Part model, mm, in its own coordinate system. Face numbers are marked on the shaded views. A direction names the side the tool comes from. Round coordinates to 2 decimals unless told otherwise and drop trailing zeros. Write each loop counter-clockwise with the first axis right and the second up, starting at its lowest first coordinate (ties: lowest second). Pieces come first, ordered by that corner, then holes. Notation, with made-up numbers: (34.25, 60) -> (61.25, 60) arc R19 ccw to (61.25, 67) -> close; hole circle Ø9 at (86, -32.5). An arc over 180 degrees is marked (long way). Use CSV: the item, a comma, the result in double quotes. Start each with the question number.
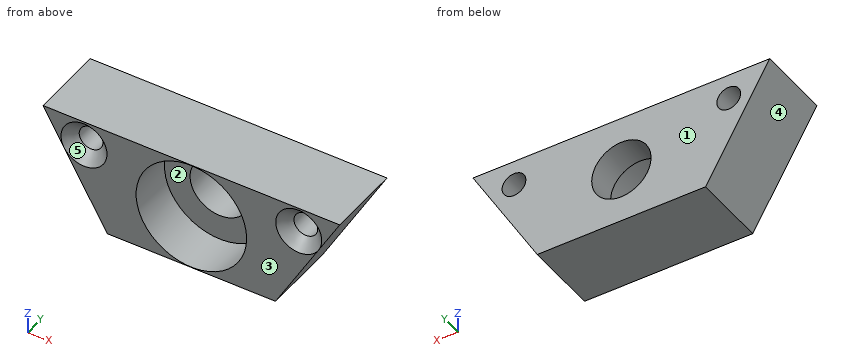
```python
from build123d import *

# Parameters (mm, degrees)
F0_R     = 1.6
F0_R_2   = 4
F1_DEPTH = 10
F2_R     = 7.45
F2_R_2   = 4
F3_DEPTH = 6


# Not quite as in the source:
# - a fillet or chamfer that OpenCascade refuses, or shapes differently, is made with other operations: its cross-section is extruded or revolved along the edge and cut away or added


with BuildPart() as f1:
    # F0 (on Front) → F1 (new body)
    with BuildSketch(Plane.XZ):
        Polygon((20, 7.5), (-20, 7.5), (-11.3397459622, -7.5), (11.3397459622, -7.5), align=None)
        with Locations((-14.4742550328, 4.1231745854)):
            Circle(F0_R, mode=Mode.SUBTRACT)
        Circle(F0_R_2, mode=Mode.SUBTRACT)
        with Locations((14.4742550328, 4.1231745854)):
            Circle(F0_R, mode=Mode.SUBTRACT)
    extrude(amount=F1_DEPTH)

    # F2 (on face) → F3 (cut)
    with BuildSketch(Plane.XZ.offset(10)):
        Circle(F2_R)
        Circle(F2_R_2, mode=Mode.SUBTRACT)
    extrude(amount=-F3_DEPTH, mode=Mode.SUBTRACT)

    # F4: chamfer of 1.5 on 2 edges, made by hand

    # F4_s1 → F4_t2 (revolve, cut)
    with BuildSketch(Plane.XY.offset(4.1231745854)):
        Polygon((-11.3742550328, -10), (-12.8742550328, -8.5), (-12.8742550328, -10), align=None)
    revolve(axis=Axis((-14.4742550328, -10, 4.1231745854), (0, -1, 0)), mode=Mode.SUBTRACT)

    # F4_s3 → F4_t4 (revolve, cut)
    with BuildSketch(Plane.XY.offset(4.1231745854)):
        Polygon((17.5742550328, -10), (16.0742550328, -8.5), (16.0742550328, -10), align=None)
    revolve(axis=Axis((14.4742550328, -10, 4.1231745854), (0, -1, 0)), mode=Mode.SUBTRACT)


solid = f1.part
```
1. Band-saw the part on C-C (z = 0). List the corners of the cut face in (x, y).
2. Pull direction Z, two halves, no side cores. Call the marked faces 3, 4 and 5: released by +Z, released by -Z, zero draft, split by the parting line, or undercut.
3. Band-saw the part on B-B (y = -1.5). List the corners of the cut face in (x, z).
4. Band-saw the part on D-D (x = 4.5). List the corners of the cut face in (y, z), then the cut area to 3 significant figures.
5. Which spindle directions (+Z, -Z, +X, -X, +Y, -Y) get a long thin tool onto all of the face, cutting with end or side? Do the marked faces 1 and 2. Say none if no direction does.
6. Flat gauge pins, fed straight in: pin 1 (3.5 mm diameter, centred on x = 14.47, z = 4.12, fed in from +Y); pin 2 (2 mm diameter, centred on x = -15.5, y = -7.5, fed in from -Z); pin 3 (4 mm diameter, centred on y = -2.5, z = 2.5, fed in from -X); pin 4 (4.5 mm diameter, centred on x = 2.5, z = 3.5, fed in from -Y). Where does each tip first touch, or does it go through?
7. Drill centre lines: line 1 along X through (y, z) = (-6.75, 5.25); line 2 along Y through (x, z) = (-6.5, 3.25); line 3 along X through (y, z) = (-1.25, 4.25). Where is each one in solid material? Low to high. Write a range as [from, to].
8. Band-saw the part on A-A (x = 0). List the corners of the cut face in (y, z).
Answers below:
1,outline,"(-15.67, -10) -> (-7.45, -10) -> (-7.45, -4) -> (-4, -4) -> (-4, 0) -> (-15.67, 0) -> close; (4, -4) -> (7.45, -4) -> (7.45, -10) -> (15.67, -10) -> (15.67, 0) -> (4, 0) -> close"
2,face 3,"zero draft"
2,face 4,"released by -Z"
2,face 5,"undercut"
3,outline,"(-20, 7.5) -> (-11.34, -7.5) -> (11.34, -7.5) -> (20, 7.5) -> close; hole circle Ø3.2 at (-14.47, 4.12); hole circle Ø8 at (0, 0); hole circle Ø3.2 at (14.47, 4.12)"
4,outline,"(-10, -7.5) -> (0, -7.5) -> (0, 7.5) -> (-10, 7.5) -> (-10, 5.94) -> (-4, 5.94) -> (-4, -5.94) -> (-10, -5.94) -> close"
4,area,"78.8 mm^2"
5,face 1,"+Z, -Z, +X, -X, +Y"
5,face 2,"-Y"
6,pin 1,"stops at y = 0"
6,pin 2,"stops at z = -2.03"
6,pin 3,"stops at x = -18.27"
6,pin 4,"stops at y = -4"
7,line 1,"x = [-18.7, -15.61], [-13.34, -5.29], [5.29, 13.34], [15.61, 18.7]"
7,line 2,"y = [-4, 0]"
7,line 3,"x = [-18.12, -16.07], [-12.88, 12.88], [16.07, 18.12]"
8,outline,"(-10, -7.5) -> (0, -7.5) -> (0, -4) -> (-4, -4) -> (-4, -7.45) -> (-10, -7.45) -> close; (-10, 7.45) -> (-4, 7.45) -> (-4, 4) -> (0, 4) -> (0, 7.5) -> (-10, 7.5) -> close"
